from build123d import *

# Parameters (mm, degrees)
SKETCH1_R           = 1
BOSS_EXTRUDE2_DEPTH = 1.6
SKETCH3_W           = 3.5
SKETCH3_H           = 8
CUT_EXTRUDE2_DEPTH  = 80.011454866
FILLET2_R           = 3
FILLET3_R           = 0.1
FILLET4_R           = 0.1
CUT_EXTRUDE3_DEPTH  = 80.011454866
LPATTERN7_COUNT     = 20
LPATTERN7_PITCH     = 2.75
FILLET5_R           = 0.5


with BuildPart() as part:
    # Sketch1 → Boss-Extrude2 (new body)
    with BuildSketch(Plane(origin=(0, 0, 0), x_dir=(1, 0, 0), z_dir=(0, 1, 0))):
        with BuildLine():
            Line((0, 0), (0, 6))
            Line((0, 6), (5.5, 71))
            ThreePointArc((5.5, 71), (7.72044875, 75.77955125), (12.5, 78))
            Line((12.5, 78), (12.5, 16.5))
            Line((12.5, 16.5), (10, 0))
            Line((10, 0), (0, 0))
        make_face()
        with Locations(Location((6.5, 4, 0), (0, 0, 270))):
            Circle(SKETCH1_R, mode=Mode.SUBTRACT)
    extrude(amount=BOSS_EXTRUDE2_DEPTH)

    # Sketch3 → Cut-Extrude2 (cut, through all)
    with BuildSketch(Plane(origin=(0, 1.6, 0), x_dir=(1, 0, 0), z_dir=(0, 1, 0))):
        with Locations((1.75, 4)):
            Rectangle(SKETCH3_W, SKETCH3_H)
    extrude(amount=-CUT_EXTRUDE2_DEPTH, mode=Mode.SUBTRACT)

    # Fillet2
    fillet2_edges = [part.edges().sort_by_distance(p)[0] for p in [
        (10, 0.8, 0),
    ]]
    fillet(fillet2_edges, radius=FILLET2_R)

    # Fillet3
    fillet3_edges = [part.edges().sort_by_distance(p)[0] for p in [
        (6.5, 0, -5),
        (6.5, 1.6, -5),
    ]]
    fillet(fillet3_edges, radius=FILLET3_R)

    # Fillet4
    fillet4_edges = [part.edges().sort_by_distance(p)[0] for p in [
        (0.169230769, 0.8, -8),
        (3.5, 0.8, -8),
        (3.5, 0.8, 0),
    ]]
    fillet(fillet4_edges, radius=FILLET4_R)

    # Sketch4 → Cut-Extrude3 (cut, through all)
    with BuildSketch(Plane(origin=(0, 1.6, 0), x_dir=(1, 0, 0), z_dir=(0, 1, 0))):
        Polygon((12.5, 73), (10.1, 72.398256348), (10.1, 71.398256348), (12.5, 70.25), align=None)
    cut_extrude3 = extrude(amount=-CUT_EXTRUDE3_DEPTH, mode=Mode.SUBTRACT)

    # LPattern7: Cut-Extrude3 ×20
    with Locations(*[(0, 0, i * LPATTERN7_PITCH) for i in range(1, LPATTERN7_COUNT)]):
        add(cut_extrude3, mode=Mode.SUBTRACT)

    # Fillet5
    fillet5_edges = [part.edges().sort_by_distance(p)[0] for p in [
        (12.5, 0.8, -78),
    ]]
    fillet(fillet5_edges, radius=FILLET5_R)


solid = part.part
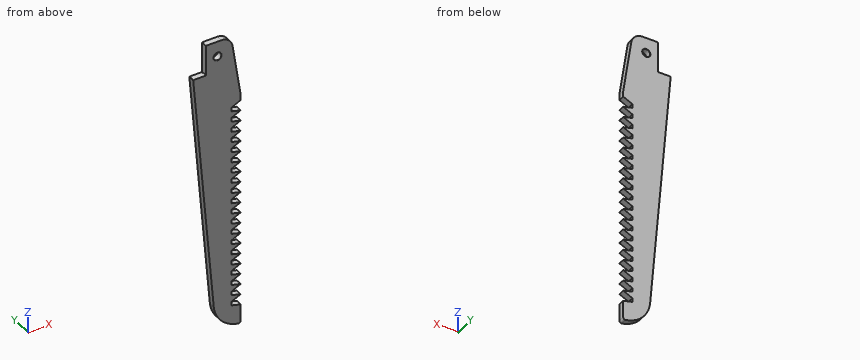
Could you check a few things on this model? Use its own coordinates, in mm. Give positions to 0.01 mm unless a question says otherwise; leave off trailing zeros. Order: outer loops, then holes, each group sorted by start corner. A loop starts at its lowest first (then second) coordinate and runs counter-clockwise, first axis right, second up. Notation, with made-up numbers: (49, -40) - (97, -40) arc R25 cw to (97, -21) - close; hole circle Ø3 at (14.5, 60.5). An arc over 180 degrees is marked (long way). One line per item, written item: value. Start each with the question number.
1. If I drill on probe 1 along X at (y, z) = (0.7, -4); probe 2 along X at (y, z) = (0.15, -19); probe 3 along Z at (x, y) = (10, 0.9), over which ranges is the centre line in solid material (lowest first)?
2. Imagine slicing it at D-D on z = -15. List the corners of the cut face in (x, y) for me, plus the area to 3 significant figures.
3. Imagine slicing it at A-A on x = 6.5. List the corners of the cut face in (y, z) for me.
4. Imagine slicing it at B-B on z = -4. List the corners of the cut face in (x, y) for me, plus the area to 3 significant figures.
5. For P1, Ø0.5, axis at y = 1, z = -72, coming from the +X side; P2, Ø0.5, axis at y = 0.5, z = -2, coming from the -X side; P3, Ø5, axis at x = 7.5, z = -49.5, coming from the -Y side, each with a flat end and sliding along its axis, tell me the tip position at first contact or that it passes through.
6. Imagine slicing it at C-C on x = 2.75. List the corners of the cut face in (y, z) for me, plus the area to 3 significant figures.
Values:
1. probe 1: 3.5 to 5.5, 7.5 to 10.61
1. probe 2: 1.1 to 10.41
1. probe 3: -77.35 to -1.47
2. outline: (0.76, 0) - (12.27, 0) - (12.27, 1.6) - (0.76, 1.6) - close
2. area: 18.4 mm²
3. outline: (0, -74.19) - (1.6, -74.19) - (1.6, -5.1) arc R0.1 ccw to (1.5, -5) - (0.1, -5) arc R0.1 ccw to (0, -5.1) - close; (0, -2.9) arc R0.1 ccw to (0.1, -3) - (1.5, -3) arc R0.1 ccw to (1.6, -2.9) - (1.6, 0) - (0, 0) - close
4. outline: (3.5, 0) - (5.4, 0) arc R0.1 ccw to (5.5, 0.1) - (5.5, 1.5) arc R0.1 ccw to (5.4, 1.6) - (3.5, 1.6) - close; (7.5, 0.1) arc R0.1 ccw to (7.6, 0) - (10.61, 0) - (10.61, 1.6) - (7.6, 1.6) arc R0.1 ccw to (7.5, 1.5) - close
4. area: 8.16 mm²
5. P1: x = 10.1
5. P2: x = 3.5
5. P3: y = 0
6. outline: (0, -38.5) - (1.6, -38.5) - (1.6, -8) - (0, -8) - close
6. area: 48.8 mm²
